```python
from build123d import *

# Parameters (mm, degrees)
CROQUIS1_R              = 16
SALIENTE_EXTRUIR1_DEPTH = 6
CROQUIS2_R              = 2.7
CROQUIS2_R_2            = 2.1
SALIENTE_EXTRUIR2_DEPTH = 5


with BuildPart() as part:
    # Croquis1 → Saliente-Extruir1 (new body)
    with BuildSketch(Plane.XY):
        Circle(CROQUIS1_R)
        with BuildLine():
            Line((2.165063509, 11.25), (1.25, 11.25))
            Line((1.25, 11.25), (1.25, 12.165063509))
            ThreePointArc((1.25, 12.165063509), (0.647047613, 12.414814566), (0, 12.5))
            ThreePointArc((0, 12.5), (-0.647047613, 12.414814566), (-1.25, 12.165063509))
            Line((-1.25, 12.165063509), (-1.25, 11.25))
            Line((-1.25, 11.25), (-2.165063509, 11.25))
            ThreePointArc((-2.165063509, 11.25), (-2.414814566, 10.647047613), (-2.5, 10))
            ThreePointArc((-2.5, 10), (-2.414814566, 9.352952387), (-2.165063509, 8.75))
            Line((-2.165063509, 8.75), (-1.25, 8.75))
            Line((-1.25, 8.75), (-1.25, 7.834936491))
            ThreePointArc((-1.25, 7.834936491), (-0.647047613, 7.585185434), (0, 7.5))
            ThreePointArc((0, 7.5), (0.647047613, 7.585185434), (1.25, 7.834936491))
            Line((1.25, 7.834936491), (1.25, 8.75))
            Line((1.25, 8.75), (2.165063509, 8.75))
            ThreePointArc((2.165063509, 8.75), (2.414814566, 9.352952387), (2.5, 10))
            ThreePointArc((2.5, 10), (2.414814566, 10.647047613), (2.165063509, 11.25))
        make_face(mode=Mode.SUBTRACT)
        with BuildLine():
            Line((11.25, -1.25), (12.165063509, -1.25))
            ThreePointArc((12.165063509, -1.25), (12.414814566, -0.647047613), (12.5, 0))
            ThreePointArc((12.5, 0), (12.414814566, 0.647047613), (12.165063509, 1.25))
            Line((12.165063509, 1.25), (11.25, 1.25))
            Line((11.25, 1.25), (11.25, 2.165063509))
            ThreePointArc((11.25, 2.165063509), (10.647047613, 2.414814566), (10, 2.5))
            ThreePointArc((10, 2.5), (9.352952387, 2.414814566), (8.75, 2.165063509))
            Line((8.75, 2.165063509), (8.75, 1.25))
            Line((8.75, 1.25), (7.834936491, 1.25))
            ThreePointArc((7.834936491, 1.25), (7.585185434, 0.647047613), (7.5, 0))
            ThreePointArc((7.5, 0), (7.585185434, -0.647047613), (7.834936491, -1.25))
            Line((7.834936491, -1.25), (8.75, -1.25))
            Line((8.75, -1.25), (8.75, -2.165063509))
            ThreePointArc((8.75, -2.165063509), (9.352952387, -2.414814566), (10, -2.5))
            ThreePointArc((10, -2.5), (10.647047613, -2.414814566), (11.25, -2.165063509))
            Line((11.25, -2.165063509), (11.25, -1.25))
        make_face(mode=Mode.SUBTRACT)
        with BuildLine():
            Line((-1.25, -11.25), (-1.25, -12.165063509))
            ThreePointArc((-1.25, -12.165063509), (-0.647047613, -12.414814566), (0, -12.5))
            ThreePointArc((0, -12.5), (0.647047613, -12.414814566), (1.25, -12.165063509))
            Line((1.25, -12.165063509), (1.25, -11.25))
            Line((1.25, -11.25), (2.165063509, -11.25))
            ThreePointArc((2.165063509, -11.25), (2.414814566, -10.647047613), (2.5, -10))
            ThreePointArc((2.5, -10), (2.414814566, -9.352952387), (2.165063509, -8.75))
            Line((2.165063509, -8.75), (1.25, -8.75))
            Line((1.25, -8.75), (1.25, -7.834936491))
            ThreePointArc((1.25, -7.834936491), (0.647047613, -7.585185434), (0, -7.5))
            ThreePointArc((0, -7.5), (-0.647047613, -7.585185434), (-1.25, -7.834936491))
            Line((-1.25, -7.834936491), (-1.25, -8.75))
            Line((-1.25, -8.75), (-2.165063509, -8.75))
            ThreePointArc((-2.165063509, -8.75), (-2.414814566, -9.352952387), (-2.5, -10))
            ThreePointArc((-2.5, -10), (-2.414814566, -10.647047613), (-2.165063509, -11.25))
            Line((-2.165063509, -11.25), (-1.25, -11.25))
        make_face(mode=Mode.SUBTRACT)
        with BuildLine():
            Line((-11.25, 1.25), (-12.165063509, 1.25))
            ThreePointArc((-12.165063509, 1.25), (-12.414814566, 0.647047613), (-12.5, 0))
            ThreePointArc((-12.5, 0), (-12.414814566, -0.647047613), (-12.165063509, -1.25))
            Line((-12.165063509, -1.25), (-11.25, -1.25))
            Line((-11.25, -1.25), (-11.25, -2.165063509))
            ThreePointArc((-11.25, -2.165063509), (-10.647047613, -2.414814566), (-10, -2.5))
            ThreePointArc((-10, -2.5), (-9.352952387, -2.414814566), (-8.75, -2.165063509))
            Line((-8.75, -2.165063509), (-8.75, -1.25))
            Line((-8.75, -1.25), (-7.834936491, -1.25))
            ThreePointArc((-7.834936491, -1.25), (-7.585185434, -0.647047613), (-7.5, 0))
            ThreePointArc((-7.5, 0), (-7.585185434, 0.647047613), (-7.834936491, 1.25))
            Line((-7.834936491, 1.25), (-8.75, 1.25))
            Line((-8.75, 1.25), (-8.75, 2.165063509))
            ThreePointArc((-8.75, 2.165063509), (-9.352952387, 2.414814566), (-10, 2.5))
            ThreePointArc((-10, 2.5), (-10.647047613, 2.414814566), (-11.25, 2.165063509))
            Line((-11.25, 2.165063509), (-11.25, 1.25))
        make_face(mode=Mode.SUBTRACT)
    extrude(amount=SALIENTE_EXTRUIR1_DEPTH)

    # Croquis2 → Saliente-Extruir2 (add)
    with BuildSketch(Plane.XY.offset(6)):
        Circle(CROQUIS2_R)
        Circle(CROQUIS2_R_2, mode=Mode.SUBTRACT)
    extrude(amount=SALIENTE_EXTRUIR2_DEPTH)


solid = part.part
```
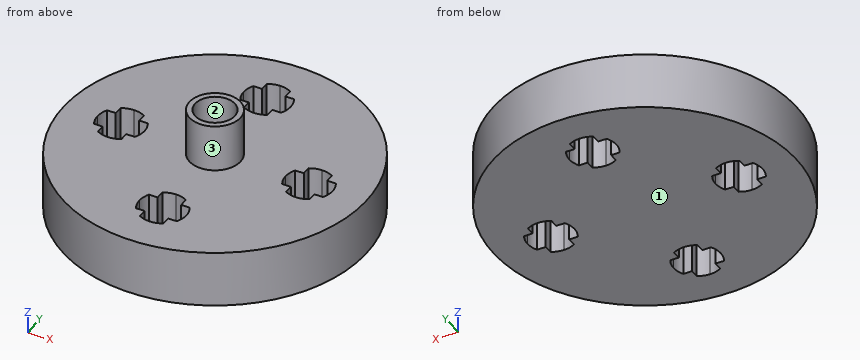
Geometry check sheet. Reference: the model listing, model coordinates, mm. Face numbers are marked on the shaded views. Give positions to 0.01 mm unless a question says otherwise; leave off trailing zeros. Loops run counter-clockwise (first coordinate to the right, second up) from the corner with the lowest first, then second, coordinate; pieces in that order, holes last. Notation, with made-up numbers: M 88.5,67 L 125.5,67 A30 cw 125.5,96 Z; hole C -16.5,72 d4. An arc over 180 degrees is marked long. Answer as CSV lines item,"result".
Item 1: Material ranges on line 1 (Y direction, x = 0, z = 9.65); line 2 (Z direction, x = 2, y = -5); line 3 (X direction, y = -10.5, z = 3), recorded low to high.
Values:
line 1,"y = -2.7 to -2.1, 2.1 to 2.7"
line 2,"z = 0 to 6"
line 3,"x = -12.07 to -2.45, 2.45 to 12.07"
Item 2: Cross-section at D-D on x = -7. Record the cut outline in (y, z).
Values:
outline,"M -14.39,0 L 14.39,0 L 14.39,6 L -14.39,6 Z"
Item 3: Cross-section at B-B on z = 2.5. Count the separate pieces of the cut face and the enclosed holes in it, and give its area (3 significant figures).
Values:
separate pieces,"1"
enclosed holes,"4"
area,"734 mm²"
Item 4: Depth check by flat-ended pin: P1, Ø3, axis at x = -6.5, z = 4.5, coming from the +Y side; P2, Ø0.7, axis at x = 8, z = 1.5, coming from the -Y side; P3, Ø1, axis at y = 1.5, z = 4, coming from the +X side; P4, Ø1, axis at x = -8, z = 7.5, coming from the +Y side. Enter the tip coordinate at first touch or a pass-through.
Values:
P1,"stops at y = 15.2"
P2,"stops at y = -14.05"
P3,"stops at x = 15.97"
P4,"passes through"
Item 5: Release check for a two-part mould opening along X. For the marked faces 1, 2 and 3 record: pulls with the +X half, pulls with the -X half, needs draft (parallel to the pull), parting line crosses it, or undercut.
Values:
face 1,"needs draft"
face 2,"undercut"
face 3,"parting line crosses it"
Item 6: Cross-section at A-A on z = 6.5. Record the cut outline in (x, y), and give its area (3 significant figures).
Values:
outline,"C 0,0 d5.4; hole C 0,0 d4.2"
area,"9.05 mm²"
Item 7: Cross-section at C-C on y = 13.5. Record the cut outline in (x, z), and give its area (3 significant figures).
Values:
outline,"M -8.59,0 L 8.59,0 L 8.59,6 L -8.59,6 Z"
area,"103 mm²"
